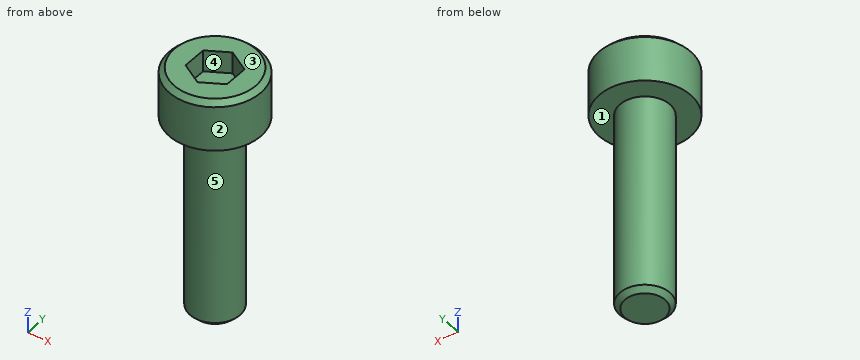
from build123d import *

# Parameters (mm, degrees)
F2_R      = 1.5
F3_DEPTH  = 12
F2_R_2    = 2.75
F3_FACE_R = 1.5
F4_DEPTH  = 3
F5_SIZE   = 0.3
F7_DEPTH  = 1.3


with BuildPart() as f3:
    # F2 (on Top) → F3 (new body)
    with BuildSketch(Plane.XY):
        Circle(F2_R)
    extrude(amount=-F3_DEPTH)

    # F2 (on Top) + F3_face (on face) → F4 (join)
    with BuildSketch(Plane.XY):
        Circle(F2_R_2)
        Circle(F2_R, mode=Mode.SUBTRACT)
    with BuildSketch(Plane.XY):
        Circle(F3_FACE_R)
    extrude(amount=F4_DEPTH)

    # F5
    f5_edges = [f3.edges().sort_by_distance(p)[0] for p in [
        (-1.5, 0, -12),
        (-2.75, 0, 3),
    ]]
    chamfer(f5_edges, length=F5_SIZE)

    # F6 (on face) → F7 (cut)
    with BuildSketch(Plane.XY.offset(3)):
        Polygon((1.25, -0.7216878365), (1.25, 0.7216878365), (0, 1.443375673), (-1.25, 0.7216878365), (-1.25, -0.7216878365), (0, -1.443375673), align=None)
    extrude(amount=-F7_DEPTH, mode=Mode.SUBTRACT)


solid = f3.part
The model under review builds one solid part; all positions refer to its coordinate system, in mm. Face numbers are marked on the shaded views. A direction names the side the tool comes from. Give positions to 0.01 mm unless a question says otherwise; leave off trailing zeros. Write each loop counter-clockwise with the first axis right and the second up, starting at its lowest first coordinate (ties: lowest second). Pieces come first, ordered by that corner, then holes.
1. Add section B-B, the plane z = -3. Write out the cut boundary in (x, y).
2. Wall thickness on L1, parallel to Z at x = -1.7, y = -1.7; L2, parallel to Z at x = -0.1, y = -0.6; L3, parallel to Y at x = -2.25, z = 2: over which ranges is each line inside the solid? List them lowest first.
3. Draft analysis for pull direction X (two halves, no side actions). For the marked faces 3, 4 and 5, state which applies: +X half, -X half, draft (parallel to the pull), parting line (faces both ways), or undercut.
4. Add section C-C, the plane z = 1. Write out the cut boundary in (x, y), plus the area to 3 significant figures.
5. For P1, Ø1.5, axis at y = 1, z = -8.5, coming from the +X side; P2, Ø1.5, axis at x = 1.5, y = -2, coming from the -Z side; P3, Ø1.2, axis at x = -0.5, y = 0.5, coming from the +Z side; P4, Ø1.5, axis at y = -1.5, z = -10.5, coming from the +X side, all flat-tipped, find the tip position at first contact; note any pin that passes through.
6. Add section A-A, the plane y = 0. Write out the cut boundary in (x, z), plus the area to 3 significant figures.
7. Tool access review of the marked faces 1 and 2: name each direction out of +Z, -Z, +X, -X, +Y, -Y from which nothing blocks a thin tool from reaching the whole face with its end or side.
Worked answers:
1. outline: circle Ø3 at (0, 0)
2. L1: z = 0 to 3
2. L2: z = -12 to 1.7
2. L3: y = -1.58 to 1.58
3. face 3: draft
3. face 4: undercut
3. face 5: parting line
4. outline: circle Ø5.5 at (0, 0)
4. area: 23.8 mm2
5. P1: stops at x = 1.48
5. P2: stops at z = 0
5. P3: stops at z = 3
5. P4: stops at x = 1.3
6. outline: (-2.75, 0) - (-1.5, 0) - (-1.5, -11.7) - (-1.2, -12) - (1.2, -12) - (1.5, -11.7) - (1.5, 0) - (2.75, 0) - (2.75, 2.7) - (2.45, 3) - (1.25, 3) - (1.25, 1.7) - (-1.25, 1.7) - (-1.25, 3) - (-2.45, 3) - (-2.75, 2.7) - close
6. area: 49.1 mm2
7. face 1: -Z
7. face 2: +Z, -Z
